Check sheet for the drawn part. Datum: minimum x, y, z corner. Units: mm. A direction names the side the tool comes from. Give positions to 0.01 mm unless a question says otherwise; leave off trailing zeros. Order: outer loops, then holes, each group sorted by start corner. A loop starts at its lowest first (then second) coordinate and runs counter-clockwise, first axis right, second up.
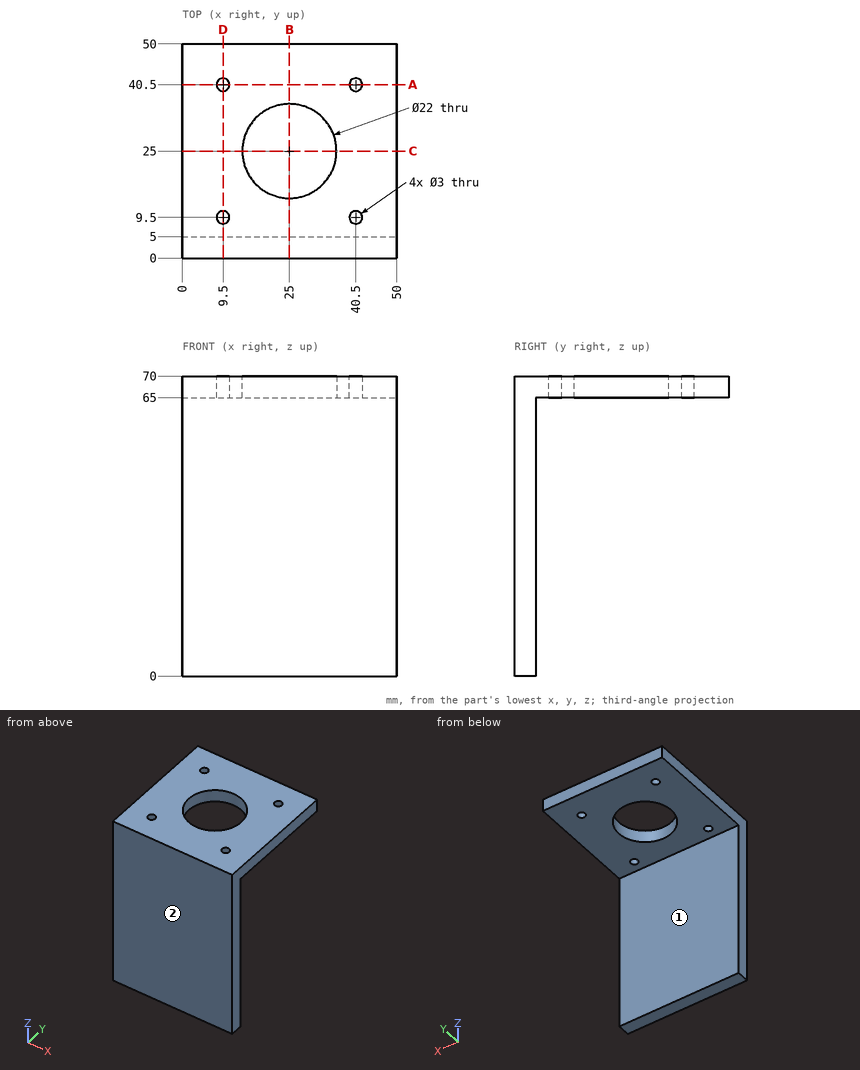
Q1. Sectioned sample at D-D, the plane x = 9.5. Record the cut outline in (y, z).
Q2. Material ranges on line 1 (Y direction, x = 9.5, z = 67.15); line 2 (X direction, y = 9, z = 66); line 3 (Y direction, x = 25, z = 68.6), recorded low to high.
Q3. Go/stop test with flat-tipped pins: P1, Ø15, axis at x = 18, z = 19.5, coming from the +Y side; P2, Ø4, axis at x = 42, y = 44, coming from the -Z side; P3, Ø3, axis at x = 36.5, z = 45, coming from the -Y side. Record where each tip stops, or that it passes through.
Q4. Sectioned sample at B-B, the plane x = 25. Record the cut outline in (y, z).
Q5. Sectioned sample at A-A, the plane y = 40.5. Record the cut outline in (x, z).
Q6. Tool access check on the marked faces 1 and 2. Record the directions out of +Z, -Z, +X, -X, +Y, -Y that give a thin tool (end or side, any length) a straight path to the whole face; none if there is none.
Q7. Sectioned sample at C-C, the plane y = 25. Record the cut outline in (x, z).
Filled in:
1. outline: (0, 0) - (5, 0) - (5, 65) - (8, 65) - (8, 70) - (0, 70) - close; (11, 65) - (39, 65) - (39, 70) - (11, 70) - close; (42, 65) - (50, 65) - (50, 70) - (42, 70) - close
2. line 1: y = 0 to 8, 11 to 39, 42 to 50
2. line 2: x = 0 to 8.09, 10.91 to 39.09, 41.91 to 50
2. line 3: y = 0 to 14, 36 to 50
3. P1: stops at y = 5
3. P2: stops at z = 65
3. P3: stops at y = 0
4. outline: (0, 0) - (5, 0) - (5, 65) - (14, 65) - (14, 70) - (0, 70) - close; (36, 65) - (50, 65) - (50, 70) - (36, 70) - close
5. outline: (0, 65) - (8, 65) - (8, 70) - (0, 70) - close; (11, 65) - (39, 65) - (39, 70) - (11, 70) - close; (42, 65) - (50, 65) - (50, 70) - (42, 70) - close
6. face 1: -Z, +X, -X, +Y
6. face 2: +Z, -Z, +X, -X, -Y
7. outline: (0, 65) - (14, 65) - (14, 70) - (0, 70) - close; (36, 65) - (50, 65) - (50, 70) - (36, 70) - close
